from build123d import *

# Parameters (mm, degrees)
SKETCH1_W               = 200
SKETCH1_H               = 120
BOSS_EXTRUDE1_DEPTH     = 10
SKETCH2_W               = 200
SKETCH2_H               = 15
BOSS_EXTRUDE2_DEPTH     = 8
SKETCH3_R               = 5
CUT_EXTRUDE1_DEPTH      = 118.046999107
SKETCH4_W               = 200
SKETCH4_H               = 23
BOSS_EXTRUDE4_DEPTH     = 16
CUT_EXTRUDE2_DEPTH      = 118.711511756
CUT_EXTRUDE2_DEPTH_BACK = 118.711511756
SKETCH3_2_R             = 5


with BuildPart() as part:
    # Sketch1 → Boss-Extrude1 (new body)
    with BuildSketch(Plane(origin=(0, 0, 0), x_dir=(1, 0, 0), z_dir=(0, 1, 0))):
        Rectangle(SKETCH1_W, SKETCH1_H)
    extrude(amount=BOSS_EXTRUDE1_DEPTH)

    # Sketch2 → Boss-Extrude2 (add)
    with BuildSketch(Plane(origin=(0, 10, 0), x_dir=(1, 0, 0), z_dir=(0, 1, 0))):
        with Locations((0, 26.999)):
            Rectangle(SKETCH2_W, SKETCH2_H)
        with Locations((0, -26.999)):
            Rectangle(SKETCH2_W, SKETCH2_H)
    extrude(amount=BOSS_EXTRUDE2_DEPTH)

    # Sketch3 → Cut-Extrude1 (cut, through all)
    with BuildSketch(Plane(origin=(0, 10, 0), x_dir=(1, 0, 0), z_dir=(0, 1, 0))):
        with Locations(Location((0, 0, 0), (0, 0, 270))):
            Circle(SKETCH3_R)
    extrude(amount=-CUT_EXTRUDE1_DEPTH, mode=Mode.SUBTRACT)

    # Sketch4 → Boss-Extrude4 (add)
    with BuildSketch(Plane(origin=(0, 10, 0), x_dir=(1, 0, 0), z_dir=(0, 1, 0))):
        Rectangle(SKETCH4_W, SKETCH4_H)
    extrude(amount=BOSS_EXTRUDE4_DEPTH)

    # Sketch3_2 → Cut-Extrude2 (cut, two sides: drawn at the far end of the back side and taken through both)
    with BuildSketch(Plane(origin=(0, 10, 0), x_dir=(1, 0, 0), z_dir=(0, 1, 0)).offset(-CUT_EXTRUDE2_DEPTH_BACK)):
        with Locations(Location((0, 0, 0), (0, 0, 270))):
            Circle(SKETCH3_2_R)
    extrude(amount=CUT_EXTRUDE2_DEPTH + CUT_EXTRUDE2_DEPTH_BACK, mode=Mode.SUBTRACT)


solid = part.part
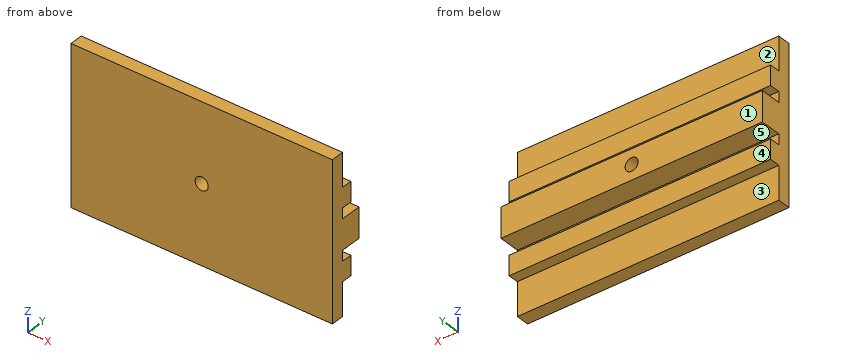
Build history of the part. All positions in model axes, mm. Face numbers are marked on the shaded views. A direction names the side the tool comes from. Round coordinates to 2 decimals unless told otherwise and drop trailing zeros. Write each loop counter-clockwise with the first axis right and the second up, starting at its lowest first coordinate (ties: lowest second). Pieces come first, ordered by that corner, then holes. Notation, with made-up numbers: M 62.25,25 L 83.25,25 A16 ccw 83.25,36 Z; hole C 63.25,-37 d5. An arc over 180 degrees is marked long. Answer as a JSON object with one key per item and string values. Group by question number.
(1) Drill centre lines: L1, parallel to Z at x = 0, y = 17; L2, parallel to Z at x = -60, y = 17; L3, parallel to X at y = 15.5, z = 0. Where is each one in solid material? Low to high.
(2) Mould opens along Z. For the marked faces 4 and 5 say: pulls with the +Z half, pulls with the -Z half, needs draft (parallel to the pull), parting line crosses it, or undercut.
(3) Which spindle directions (+Z, -Z, +X, -X, +Y, -Y) get a long thin tool onto all of the face, cutting with end or side? Do the marked faces 1, 2 and 3. Say none if no direction does.
(4) Cut at C-C (z = 0). Give the cut face in (x, y), and give its area (3 significant figures).
(5) Cut at D-D (x = 34). Give the cut face in (y, z).
(6) Cut at A-A (x = 0). Give the cut face in (y, z), and give its area (3 significant figures).
(7) Flat gauge pins, fed straight in: pin 1 (20.5 mm diameter, centred on x = -49, z = -45.5, fed in from +Y); pin 2 (4 mm diameter, centred on x = 19.5, y = 14.5, fed in from +Z); pin 3 (1 mm diameter, centred on x = -25.5, z = 23, fed in from +Y). Where does each tip first touch, or does it go through?
(8) Cut at B-B (y = 13.5). Give the cut face in (x, z).
Responses:
{
 "1": {"L1": "z = -34.5 to -19.5, -11.5 to -5, 5 to 11.5, 19.5 to 34.5", "L2": "z = -34.5 to -19.5, -11.5 to 11.5, 19.5 to 34.5", "L3": "x = -100 to -5, 5 to 100"},
 "2": {"face 4": "needs draft", "face 5": "undercut"},
 "3": {"face 1": "+Z, -Z, +X, -X, +Y", "face 2": "+Z, +X, -X, +Y", "face 3": "-Z, +X, -X, +Y"},
 "4": {"outline": "M -100,0 L -5,0 L -5,26 L -100,26 Z; M 5,0 L 100,0 L 100,26 L 5,26 Z", "area": "4,940 mm2"},
 "5": {"outline": "M 0,-60 L 10,-60 L 10,-34.5 L 18,-34.5 L 18,-19.5 L 10,-19.5 L 10,-11.5 L 26,-11.5 L 26,11.5 L 10,11.5 L 10,19.5 L 18,19.5 L 18,34.5 L 10,34.5 L 10,60 L 0,60 Z"},
 "6": {"outline": "M 0,-60 L 10,-60 L 10,-34.5 L 18,-34.5 L 18,-19.5 L 10,-19.5 L 10,-11.5 L 26,-11.5 L 26,-5 L 0,-5 Z; M 0,5 L 26,5 L 26,11.5 L 10,11.5 L 10,19.5 L 18,19.5 L 18,34.5 L 10,34.5 L 10,60 L 0,60 Z", "area": "1,550 mm2"},
 "7": {"pin 1": "stops at y = 10", "pin 2": "stops at z = 34.5", "pin 3": "stops at y = 18"},
 "8": {"outline": "M -100,-34.5 L 100,-34.5 L 100,-19.5 L -100,-19.5 Z; M -100,-11.5 L 100,-11.5 L 100,11.5 L -100,11.5 Z; M -100,19.5 L 100,19.5 L 100,34.5 L -100,34.5 Z; hole C 0,0 d10"}
}
